Part model, mm, in its own coordinate system. A direction names the side the tool comes from. Round coordinates to 2 decimals unless told otherwise and drop trailing zeros. Loops run counter-clockwise (first coordinate to the right, second up) from the corner with the lowest first, then second, coordinate; pieces in that order, holes last. Notation, with made-up numbers: M -18,65.25 L -6,65.25 A19 cw -6,71.25 Z; hole C -15.5,2 d8. An arc over 180 degrees is marked long. Answer as CSV lines item,"result". Start each with the question number.
Item 1: Band-saw the part on B-B (y = -35.5). Give the cut face in (x, z), and give its area (3 significant figures).
Item 2: Band-saw the part on C-C (x = -42). Give the cut face in (y, z).
Item 3: Band-saw the part on D-D (z = -35). Give the cut face in (x, y).
Item 4: Drop flat-ended pins along their axis: pin 1 Ø6 at (x, y) = (30, -130.5) entering from -Z; pin 2 Ø10 at (x, z) = (-5, -55.5) entering from -Y; pin 3 Ø10 at (x, z) = (-9.5, 42) entering from -Y. Give the stop position or say it passes through.
Item 5: Mould opens along X. For faces 1 (the flat face through (0, -145, -54)), 2 (the flat face through (0, -81, -39.278)), 3 (the flat face through (-24.37, -140, -54)) say: pulls with the +X half, pulls with the -X half, needs draft (parallel to the pull), parting line crosses it, or undercut.
Item 6: Wall check: line 1 (Z direction, x = 25, y = -42); line 2 (X direction, y = -136, z = 43); line 3 (Y direction, x = -3, z = 7). Give the ranges that are in metal, low to high.
Item 7: Which spindle directions (+Z, -Z, +X, -X, +Y, -Y) get a long thin tool onto all of the face, cutting with end or side? Do faces 4 (the flat face through (0, -81, 50.722)), 5 (the flat face through (-24.37, -95, -54)), 6 (the flat face through (25.63, -140, -54)), 7 (the flat face through (0, -100, -54)). Say none if no direction does.
Item 8: Band-saw the part on A-A (z = -53.5). Give the cut face in (x, y).
```python
from build123d import *

# Parameters (mm, degrees)
F0_W     = 100
F0_H     = 100
F1_DEPTH = 150
F2_W     = 90
F2_H     = 90
F3_DEPTH = 140
F4_W     = 50
F4_H     = 10
F5_DEPTH = 20


with BuildPart() as f1:
    # F0 (on Front) → F1 (new body)
    with BuildSketch(Plane.XZ):
        with Locations((0.630199, 5.721866)):
            Rectangle(F0_W, F0_H)
    extrude(amount=F1_DEPTH)

    # F2 (on face) → F3 (cut)
    with BuildSketch(Plane.XZ.offset(150)):
        with Locations((0.630199, 5.721866)):
            Rectangle(F2_W, F2_H)
    extrude(amount=-F3_DEPTH, mode=Mode.SUBTRACT)

    # F4 (on face) → F5 (join)
    with BuildSketch(Plane(origin=(0, 0, -44.278134), x_dir=(1, 0, 0), z_dir=(0, 0, -1))):
        with Locations((0.630199, 140)):
            Rectangle(F4_W, F4_H)
        with Locations((0.630199, 95)):
            Rectangle(F4_W, F4_H)
    extrude(amount=F5_DEPTH)


solid = f1.part
```
Answer block:
1,outline,"M -49.37,-44.28 L 50.63,-44.28 L 50.63,55.72 L -49.37,55.72 Z; hole M -44.37,-39.28 L 45.63,-39.28 L 45.63,50.72 L -44.37,50.72 Z"
1,area,"1,900 mm^2"
2,outline,"M -150,-44.28 L 0,-44.28 L 0,55.72 L -150,55.72 L -150,50.72 L -10,50.72 L -10,-39.28 L -150,-39.28 Z"
3,outline,"M -49.37,-150 L -44.37,-150 L -44.37,-10 L 45.63,-10 L 45.63,-150 L 50.63,-150 L 50.63,0 L -49.37,0 Z"
4,pin 1,"stops at z = -44.28"
4,pin 2,"stops at y = -145"
4,pin 3,"stops at y = -10"
5,face 1,"needs draft"
5,face 2,"undercut"
5,face 3,"pulls with the -X half"
6,line 1,"z = -44.28 to -39.28, 50.72 to 55.72"
6,line 2,"x = -49.37 to -44.37, 45.63 to 50.63"
6,line 3,"y = -10 to 0"
7,face 4,"-Y"
7,face 5,"-Z, -X, +Y, -Y"
7,face 6,"-Z, +X, +Y, -Y"
7,face 7,"-Z, +X, -X"
8,outline,"M -24.37,-145 L 25.63,-145 L 25.63,-135 L -24.37,-135 Z; M -24.37,-100 L 25.63,-100 L 25.63,-90 L -24.37,-90 Z"
